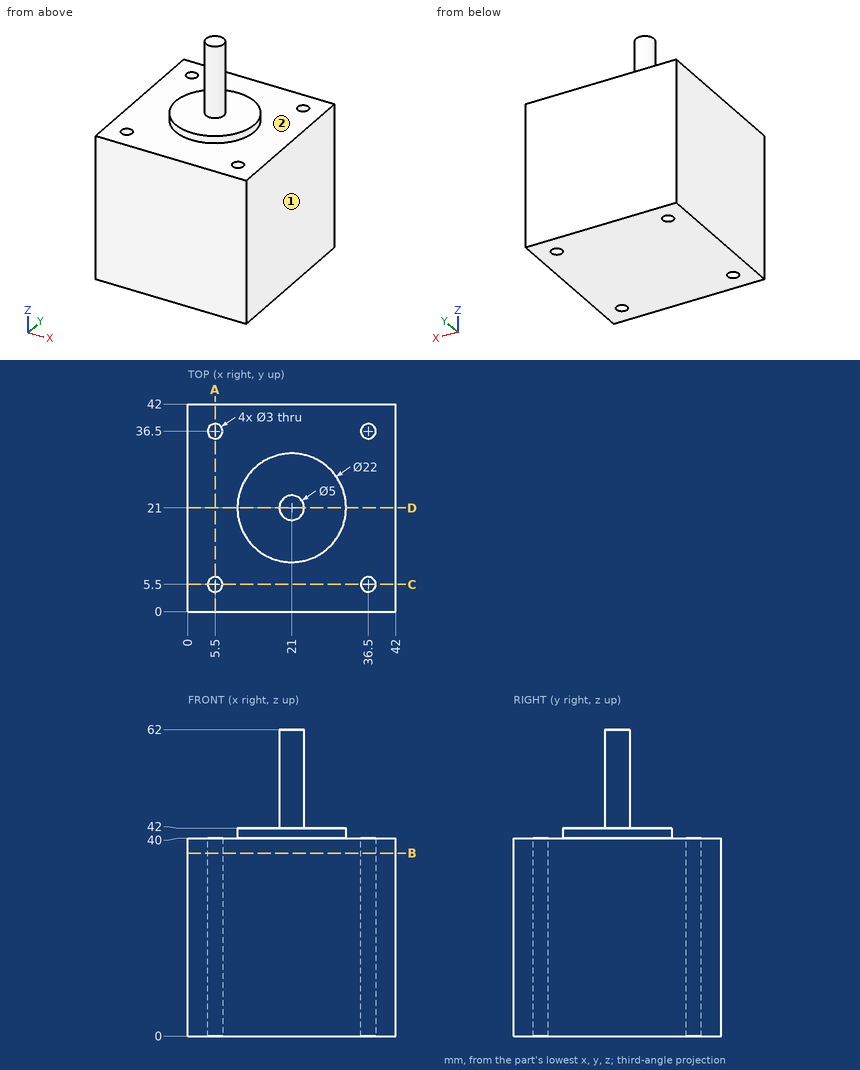
Job drawing, mm, ordinate dimensions from the low corner. One solid piece. A direction names the side the tool comes from. Coordinates: 2 decimals unless noted, no trailing zeros. Order: outer loops, then holes, each group sorted by start corner. A loop starts at its lowest first (then second) coordinate and runs counter-clockwise, first axis right, second up. Notation, with made-up numbers: (9.5, 76) -> (33.5, 76) arc R25 ccw to (33.5, 92) -> close; hole circle Ø4 at (38, 2.5). An arc over 180 degrees is marked (long way). Put each result on its own line as item: value. Start each with the question number.
(1) Band-saw the part on D-D (y = 21). Give the cut face in (x, z).
(2) Probe line 1 along Y through (x, z) = (36.5, 11); line 2 along Y through (x, z) = (6, 31). List the from-to ranges inside material, lowest first. Write a range as [from, to].
(3) Pin check, flat tips, straight feed: pin 1 Ø12 at (x, z) = (26.5, 16.5) entering from -Y; pin 2 Ø1.8 at (x, y) = (36.5, 5.5) entering from +Z; pin 3 Ø1 at (y, z) = (18.5, 45) entering from +X; pin 4 Ø1 at (x, y) = (31.5, 7.5) entering from +Z. Stop position of each tip, or through.
(4) Band-saw the part on B-B (z = 37). Give the cut face in (x, y).
(5) Which spindle directions (+Z, -Z, +X, -X, +Y, -Y) get a long thin tool onto all of the face, cutting with end or side? Do the marked faces 1 and 2. Say none if no direction does.
(6) Band-saw the part on A-A (x = 5.5). Give the cut face in (y, z).
Determined:
1. outline: (0, 0) -> (42, 0) -> (42, 40) -> (32, 40) -> (32, 42) -> (23.5, 42) -> (23.5, 62) -> (18.5, 62) -> (18.5, 42) -> (10, 42) -> (10, 40) -> (0, 40) -> close
2. line 1: y = [0, 4], [7, 35], [38, 42]
2. line 2: y = [0, 4.09], [6.91, 35.09], [37.91, 42]
3. pin 1: stops at y = 0
3. pin 2: passes through
3. pin 3: stops at x = 22.5
3. pin 4: stops at z = 40
4. outline: (0, 0) -> (42, 0) -> (42, 42) -> (0, 42) -> close; hole circle Ø3 at (5.5, 5.5); hole circle Ø3 at (5.5, 36.5); hole circle Ø3 at (36.5, 5.5); hole circle Ø3 at (36.5, 36.5)
5. face 1: +Z, -Z, +X, +Y, -Y
5. face 2: +Z
6. outline: (0, 0) -> (4, 0) -> (4, 40) -> (0, 40) -> close; (7, 0) -> (35, 0) -> (35, 40) -> (7, 40) -> close; (38, 0) -> (42, 0) -> (42, 40) -> (38, 40) -> close
